Can you work these out from the model? Positions are in its coordinate system, mm. Face numbers are marked on the shaded views. Coordinates: 2 decimals unless noted, no trailing zeros. Loops run counter-clockwise (first coordinate to the right, second up) from the corner with the lowest first, then second, coordinate; pieces in that order, holes last. Notation, with made-up numbers: (18, 48.5) - (53, 48.5) arc R19 cw to (53, 82.5) - close; hole circle Ø2 at (27, 14). An arc over 180 degrees is marked (long way). Put each result on its own line as item: value. Start each with the question number.
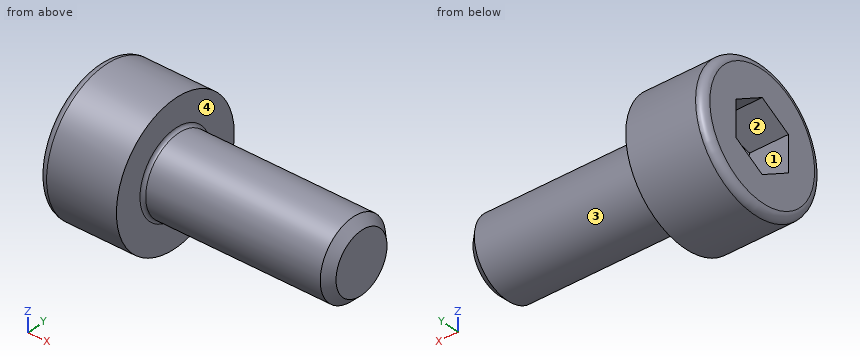
Autodesk Inventor part; units mm, degrees
ref_plane "Work Plane1" through (29, 0, 0) normal (0, -1, 0) x (1, 0, 0)
ref_plane "YZ Plane" through (0, 0, 0) normal (1, 0, 0) x (0, 1, 0)
ref_plane "XZ Plane" through (0, 0, 0) normal (0, 1, 0) x (-1, 0, 0)
sketch "Sketch1" plane through (0, 0, 0) normal (0, 0, 1) x (1, 0, 0)
  line L0 (-0.5833, 0) -> (6, 0)
  line L1 (6, 0) -> (6, 1.25)
  line L2 (6, 1.25) -> (1.1761, 1.25)
  line L3 (1.1761, 1.25) -> (0.8999, 1.25)
  line L4 (0.8999, 1.25) -> (0, 1.25)
  line L5 (0, 1.25) -> (0, 2.25)
  line L6 (0, 2.25) -> (-2.5, 2.25)
  line L7 (-2.5, 2.25) -> (-2.5, 1.1547)
  line L8 (-2.5, 1.1547) -> (-1.25, 1.1547)
  line L9 (-1.25, 1.1547) -> (-0.5833, 0)
  line L10 (-4.2, 0) -> (7.7, 0)
  line L11 (0, -0.45) -> (0, 2.7)
  line L12 (1.1761, 1.25) -> (0, 1.25) construction
  dimension "d1" = 4.8239
  dimension "d2" = 0.2762
  dimension "d3" = 2.5
  dimension "d4" = 1.25
  dimension "d5" = 60
  dimension "d6" = 2.5
  dimension "d7" = 2.5
  dimension "d8" = 2.3094
  dimension "d9" = 4.5
  dimension "d26" = 6
revolve "Body" add sketch "Sketch1" angle 360 about axis through (-0.5833, 0, 0) along (1, 0, 0)
sketch "Sketch2" plane through (-2.5, 0, 0) normal (-1, 0, 0) x (0, 0, 1)
  circle A0 centre (0, 0) radius 1.1547
  line L0 (0, -3.15) -> (0, 3.15)
  line L1 (-3.15, 0) -> (3.15, 0)
  line L2 (1.1547, 0) -> (0.5774, -1)
  line L3 (0.5774, -1) -> (-0.5774, -1)
  line L4 (-0.5774, -1) -> (-1.1547, 0)
  line L5 (-1.1547, 0) -> (-0.5774, 1)
  line L6 (-0.5774, 1) -> (0.5774, 1)
  line L7 (0.5774, 1) -> (1.1547, 0)
extrude "Slot" add sketch "Sketch2" against normal up to next contours L7 A0 | A0 L2 | L6 L0 A0 | A0 L0 L3 | L0 L6 A0 | A0 L3 L0 | L4 A0 | A0 L5
fillet "Fillet1" radius 0.25 1 edges at (-2.5, -2.25, 0)
thread "Thread"
chamfer "Chamfer1" distance 0.2761 distance2 0.2761 1 edges at (6, -1.25, 0) measured on face at (6, -0.1825, -0.5629)
ref_plane "Work Plane1" through (29, 0, 0) normal (0, -1, 0) x (1, 0, 0)
fillet "Fillet2" radius 0.1 1 edges at (0, -1.25, 0)
equation "\"d30\" = R"
equation "\"d17\" = RR"
equation "\"d13\" = GEL"
equation "\"d15\" = -0.5 * SPD + 0.5 * GD"
equation "\"d16\" = GUL"
equation "\"d1\" = GEL"
equation "\"d3\" = KOH"
equation "\"d4\" = INTI"
equation "\"d6\" = GD"
equation "\"d7\" = BDM"
equation "\"d8\" = 1.1547 * SW"
equation "\"d9\" = KOD"
equation "\"d26\" = NLG"
equation "\"GD\" = NND"
equation "\"NLG\" = 6"
equation "\"GEL\" = 4.82395"
equation "\"KOD\" = 4.5"
equation "\"KOH\" = 2.5"
equation "\"INTI\" = 1.25"
equation "\"GAL\" = 0.61345 * PTC"
equation "\"GUL\" = 0.61345 * PTC"
equation "\"BDM\" = NND"
equation "\"SW\" = 2"
equation "\"RR\" = 0.25"
equation "\"SPD\" = 1.94789"
equation "\"R\" = 0.1"
equation "\"TOA\" = 30deg"
equation "\"THREADDIA\" = 2.5"
equation "\"PTC\" = 0.45"
equation "\"NND\" = 2.5"
equation "\"E0\" = 1.155 * SW"
equation "\"GD1\" = THREADDIA - 1.2269 * PTC"
properties part number "ANSI B18.3.1M - M2.5x0.45 x 6" material "Steel, Mild"
Q1. Please list where these lines run through material, in increasing order: line 1 along Z through (x, y) = (2.75, 0); line 2 along X through (y, z) = (-1.8, 0.7); line 3 along Z through (x, y) = (-1.25, 1.8). Write a range as [from, to].
Q2. I want a section at A-A on x = 1. List the corners of the cut face in (y, z) for me, and give its area (3 significant figures).
Q3. We'd pull the mould along Z, two halves only. Please class the marked faces 1, 2, 3 and 4: released by +Z, released by -Z, zero draft, split by the parting line, or undercut.
Q4. Will these pins go through, and if not, where does the flat tip stop? pin 1 (1 mm diameter, centred on x = 0, y = 1.5, fed in from -Z); pin 2 (1.5 mm diameter, centred on x = 3.5, y = 0.5, fed in from +Z).
Calculated:
1. line 1: [-1.25, 1.25]
1. line 2: [-2.5, 0]
1. line 3: [-1.35, 1.35]
2. outline: circle Ø2.5 at (0, 0)
2. area: 4.91 mm2
3. face 1: undercut
3. face 2: undercut
3. face 3: split by the parting line
3. face 4: zero draft
4. pin 1: z = -2.02
4. pin 2: z = 1.25
